CAD build for the part. Positions are in the model's coordinates, mm. Face numbers are marked on the shaded views. A direction names the side the tool comes from. Give positions to 0.01 mm unless a question says otherwise; leave off trailing zeros. Write each loop counter-clockwise with the first axis right and the second up, starting at its lowest first coordinate (ties: lowest second). Pieces come first, ordered by that corner, then holes. Notation, with made-up numbers: (49, 64.5) - (93, 64.5) arc R17 ccw to (93, 81.5) - close; hole circle Ø10 at (55.5, 78). An arc over 180 degrees is marked (long way). Answer as a JSON object with one key per item and string values.
from build123d import *

# Parameters (mm, degrees)
F1_DEPTH = 150
F2_R     = 2.5
F3_DEPTH = 20.001
F4_W     = 100
F4_H     = 20
F5_DEPTH = 20.001
F7_DEPTH = 25


with BuildPart() as f1:
    # F0 (on Front) → F1 (new body)
    with BuildSketch(Plane.XZ):
        Polygon((90, -90), (90, 90), (70, 90), (70, 10), (-40, 10), (-40, -40), (-90, -40), (-90, -90), align=None)
    extrude(amount=-F1_DEPTH)

    # F2 (on face) → F3 (cut, through all)
    with BuildSketch(Plane(origin=(70, 0, 0), x_dir=(0, -1, 0), z_dir=(-1, 0, 0))):
        with Locations((-75, 78.577638)):
            Circle(F2_R)
    extrude(amount=-F3_DEPTH, mode=Mode.SUBTRACT)

    # F4 (on face) → F5 (cut, through all)
    with BuildSketch(Plane(origin=(70, 0, 0), x_dir=(0, -1, 0), z_dir=(-1, 0, 0))):
        with Locations((-75, 55)):
            Rectangle(F4_W, F4_H)
    extrude(amount=-F5_DEPTH, mode=Mode.SUBTRACT)

    # F6 (on face) → F7 (cut)
    with BuildSketch(Plane.XY.offset(-40)):
        with BuildLine():
            Line((-50, 35), (-50, 115))
            ThreePointArc((-50, 115), (-65, 130), (-80, 115))
            Line((-80, 115), (-80, 35))
            ThreePointArc((-80, 35), (-65, 20), (-50, 35))
        make_face()
    extrude(amount=-F7_DEPTH, mode=Mode.SUBTRACT)


solid = f1.part
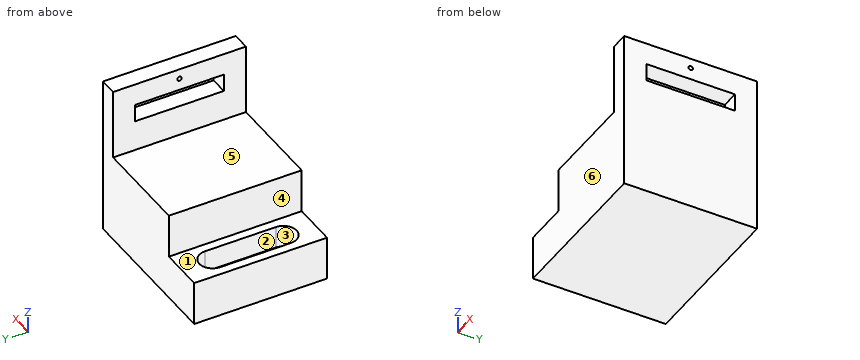
(1) Saw through at C-C, the plane y = 93.5. Give the cut face in (x, z), and give its area (4 significant figures).
Answer key:
{"outline": "(-90, -90) - (90, -90) - (90, 45) - (70, 45) - (70, 10) - (-40, 10) - (-40, -40) - (-50, -40) - (-50, -65) - (-80, -65) - (-80, -40) - (-90, -40) - close; (70, 65) - (90, 65) - (90, 90) - (70, 90) - close", "area": "15,950 mm²"}
(2) Saw through at D-D, the plane x = -65. Give the cut face in (y, z).
Answer key:
{"outline": "(0, -90) - (150, -90) - (150, -40) - (130, -40) - (130, -65) - (20, -65) - (20, -40) - (0, -40) - close"}
(3) Saw through at B-B, the plane y = 75. Give the cut face in (x, z).
Answer key:
{"outline": "(-90, -90) - (90, -90) - (90, 45) - (70, 45) - (70, 10) - (-40, 10) - (-40, -40) - (-50, -40) - (-50, -65) - (-80, -65) - (-80, -40) - (-90, -40) - close; (70, 65) - (90, 65) - (90, 76.08) - (70, 76.08) - close; (70, 81.08) - (90, 81.08) - (90, 90) - (70, 90) - close"}
(4) Flat gauge pins, fed straight in: P1, Ø4, axis at x = 12, y = 73.5, coming from the +Z side; P2, Ø5, axis at y = 62, z = 23, coming from the -X side; P3, Ø10, axis at x = -56, y = 128, coming from the +Z side; P4, Ø10, axis at x = 81.5, z = 56.5, coming from the -Y side. Where does each tip first touch, or does it go through?
Answer key:
{"P1": "stops at z = 10", "P2": "stops at x = 70", "P3": "stops at z = -40", "P4": "stops at y = 0"}
(5) Saw through at A-A, the plane z = -60.5. Give the cut face in (x, y), and give its area (3 significant figures).
Answer key:
{"outline": "(-90, 0) - (90, 0) - (90, 150) - (-90, 150) - close; hole (-80, 35) arc R15 ccw to (-50, 35) - (-50, 115) arc R15 ccw to (-80, 115) - close", "area": "23,900 mm²"}
(6) 3-axis set-ups, long thin cutter, end or side, ignore diameter. For the marked faces 5 and 6: which of +Z, -Z, +X, -X, +Y, -Y reach the whole face in a straight line?
Answer key:
{"face 5": "+Z, -X, +Y, -Y", "face 6": "+Z, -Z, +X, -X, -Y"}
(7) Pull direction X, two halves, no side cores. Call the marked faces 1, 2, 3 and 4: pulls with the +X half, pulls with the -X half, needs draft (parallel to the pull), parting line crosses it, or undercut.
Answer key:
{"face 1": "needs draft", "face 2": "undercut", "face 3": "undercut", "face 4": "pulls with the -X half"}
(8) Probe L1, parallel to Z at x = 77.5, y = 75; L2, parallel to X at y = 92, z = -63; L3, parallel to Z at x = -6, y = 128. List the from-to ranges inside material, lowest first. Write a range as [from, to].
Answer key:
{"L1": "z = [-90, 45], [65, 76.08], [81.08, 90]", "L2": "x = [-90, -80], [-50, 90]", "L3": "z = [-90, 10]"}
